The model under review builds one solid part; all positions refer to its coordinate system, in mm. A direction names the side the tool comes from. Round coordinates to 2 decimals unless told otherwise and drop trailing zeros. Order: outer loops, then holes, each group sorted by start corner. A loop starts at its lowest first (then second) coordinate and runs counter-clockwise, first axis right, second up. Notation, with made-up numbers: M 81.25,15.25 L 92.25,15.25 A22 cw 92.25,48.25 Z; hole C -32,5.25 d2. An arc over 180 degrees is marked long. Answer as a JSON object with one key per item and string values. Group by question number.
1) Insertion check: pin 1 Ø12 at (y, z) = (7.5, -22) entering from -X; pin 2 Ø1 at (x, y) = (-10.5, 7) entering from -Z; pin 3 Ø1.5 at (y, z) = (-3.5, -10.5) entering from +X. Each pin has a flat end and moves straight along its axis. Give the tip position at first contact, or say it passes through.
2) The part is to be moulded in two halves that separate along Z. For faces 1 (the flat face through (9, -12, 9)), 2 (the cylindrical face through (23.323, 6.902, 2.103)), 3 (the cylindrical face through (39.923, 7.098, -20.765)), 4 (the conical face through (10.434, 2.812, 2.317)), say which applies: +Z half, -Z half, draft (parallel to the pull), parting line (faces both ways), or undercut.
3) Consider section B-B, the plane z = -30. Write out the cut boundary in (x, y), then the cut area to 3 significant figures.
4) For faces 5 (the flat face through (3, 0, -9)), 6 (the flat face through (19, 0, 9)), 7 (the cylindrical face through (-3.2, 8.4, -10)), 8 (the cylindrical face through (-23.534, 6.902, 2.681)), 9 (the flat face through (-11, 14, 1)), list the 3-axis set-ups (+Z, -Z, +X, -X, +Y, -Y) from which the entire face can be reached by the end or side of a thin tool; tool diameter is ignored.
5) Consider section D-D, the plane x = 31.5. Write out the cut boundary in (y, z), then the cut area to 3 significant figures.
6) Consider section A-A, the plane x = 0. Count the separate pieces of the cut face and the enclosed holes in it, then the cut area to 3 significant figures.
7) Consider section C-C, the plane y = 7.75. Write out the cut boundary in (x, z).
8) To check wall thickness, follow line 1 (X direction, y = -9.5, z = 0); line 2 (Z direction, x = 2, y = 10); line 3 (Z direction, x = -4.5, y = 0.75). State the ranges of each line that lie inside material, in increasing order.
```python
from build123d import *

# Parameters (mm, degrees)
SKETCH_3_R               = 7
CUT_EXTRUDE_1_DEPTH      = 14
PATTERN_CIRCULAR_1_COUNT = 4


with BuildPart() as part:
    # 草图2 → 旋转1 (revolve)
    with BuildSketch(Plane(origin=(0, 0, 0), x_dir=(0, 0, -1), z_dir=(1, 0, 0))):
        Polygon((12, -12), (20, -12), (20, -7.5), (20, 0), (45, 0), (45, 14), (10.5, 14), (10.5, 3), (13.5, 0), (9, 0), (9, -7.5), (12, -7.5), align=None)
    revolve(axis=Axis((0, 0, 0), (0, 1, 0)))

    # 草图3 → 切除-拉伸1 (cut)
    with BuildSketch(Plane(origin=(0, 0, 0), x_dir=(1, 0, 0), z_dir=(0, 1, 0))):
        with Locations(Location((0, 30, 0), (0, 0, 270))):
            Circle(SKETCH_3_R)
    cut_extrude_1 = extrude(amount=CUT_EXTRUDE_1_DEPTH, mode=Mode.SUBTRACT)

    # 阵列(圆周)1: 切除-拉伸1 ×4 about axis
    pattern_circular_1_axis = Axis((0, 0, 0), (0, 1, 0))
    for i in range(1, PATTERN_CIRCULAR_1_COUNT):
        add(cut_extrude_1.rotate(pattern_circular_1_axis, i * 360 / PATTERN_CIRCULAR_1_COUNT), mode=Mode.SUBTRACT)


solid = part.part
```
Results list:
{
 "1": {"pin 1": "x = -42.06", "pin 2": "z = -43.87", "pin 3": "x = 17.46"},
 "2": {"face 1": "draft", "face 2": "undercut", "face 3": "parting line", "face 4": "undercut"},
 "3": {"outline": "M -33.54,0 L -7,0 L -7,14 L -33.54,14 Z; M 7,0 L 33.54,0 L 33.54,14 L 7,14 Z", "area": "743 mm^2"},
 "4": {"face 5": "none", "face 6": "-Y", "face 7": "+Y", "face 8": "+Y, -Y", "face 9": "+Z, -Z, +X, -X, +Y"},
 "5": {"outline": "M 0,-32.14 L 14,-32.14 L 14,-6.84 L 0,-6.84 Z; M 0,6.84 L 14,6.84 L 14,32.14 L 0,32.14 Z", "area": "708 mm^2"},
 "6": {"separate pieces": "4", "enclosed holes": "0", "area": "802 mm^2"},
 "7": {"outline": "C 0,0 d90; hole C -30,0 d14; hole C 0,0 d21; hole C 0,-30 d14; hole C 0,30 d14; hole C 30,0 d14"},
 "8": {"line 1": "-20 to -12, 12 to 20", "line 2": "-44.96 to -36.71, -23.29 to -10.31, 10.31 to 23.29, 36.71 to 44.96", "line 3": "-44.77 to -35.36, -24.64 to -11.93, 11.93 to 24.64, 35.36 to 44.77"}
}
